from build123d import *

# Parameters (mm, degrees)
BOSS_EXTRUDE1_DEPTH = 2.5


with BuildPart() as part:
    # Sketch1 → Boss-Extrude1 (new, symmetric)
    with BuildSketch(Plane(origin=(0, 0, 0), x_dir=(1, 0, 0), z_dir=(0, 1, 0))):
        Polygon((114, 145), (114, 150), (84, 150), (84, 145), (48, 145), (48, 150), (18, 150), (18, 145), (-18, 145), (-18, 150), (-48, 150), (-48, 145), (-84, 145), (-84, 150), (-114, 150), (-114, 145), (-140, 145), (-140, 114), (-145, 114), (-145, 84), (-140, 84), (-140, 48), (-145, 48), (-145, 18), (-140, 18), (-140, -18), (-145, -18), (-145, -48), (-140, -48), (-140, -84), (-145, -84), (-145, -114), (-140, -114), (-140, -145), (-114, -145), (-114, -150), (-84, -150), (-84, -145), (-48, -145), (-48, -150), (-18, -150), (-18, -145), (18, -145), (18, -150), (48, -150), (48, -145), (84, -145), (84, -150), (114, -150), (114, -145), (140, -145), (140, -114), (145, -114), (145, -83.328035024), (140, -83.328035024), (140, -47.328035024), (145, -47.328035024), (145, -17.328035024), (140, -17.328035024), (140, 18.671964976), (145, 18.671964976), (145, 48.671964976), (140, 48.671964976), (140, 84), (145, 84), (145, 114), (140, 114), (140, 145), align=None)
    extrude(amount=BOSS_EXTRUDE1_DEPTH, both=True)


solid = part.part
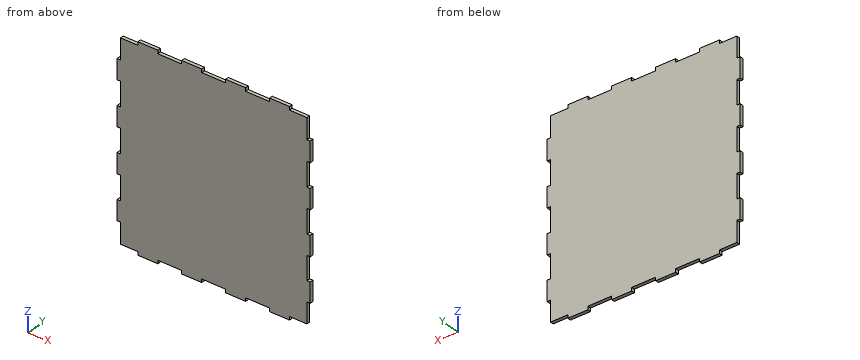
Model file for the job. Use its own axes, mm. Give positions to 0.01 mm unless a question says otherwise; leave off trailing zeros. Loops run counter-clockwise (first coordinate to the right, second up) from the corner with the lowest first, then second, coordinate; pieces in that order, holes last.
1) Flat gauge pins, fed straight in: pin 1 Ø2.5 at (x, y) = (-143.5, 0) entering from -Z; pin 2 Ø1.5 at (y, z) = (-1, 147.5) entering from +X; pin 3 Ø1.5 at (y, z) = (0.5, 129.5) entering from -X. Where does each tip first touch, or does it go through?
2) Saw through at A-A (x = 75.5). Write the cut outline in (y, z), plus the area to 3 significant figures.
3) Saw through at B-B (z = -76). Write the cut outline in (x, y).
4) Wall check: line 1 (X direction, y = -0.5, z = -82.5); line 2 (Z direction, x = 54, y = -0.65). Give the ranges that are in metal, low to high.
Answer block:
1. pin 1: stops at z = -114
1. pin 2: stops at x = 114
1. pin 3: stops at x = -140
2. outline: (-2.5, -145) - (2.5, -145) - (2.5, 145) - (-2.5, 145) - close
2. area: 1,450 mm2
3. outline: (-140, -2.5) - (140, -2.5) - (140, 2.5) - (-140, 2.5) - close
4. line 1: x = -140 to 140
4. line 2: z = -145 to 145
